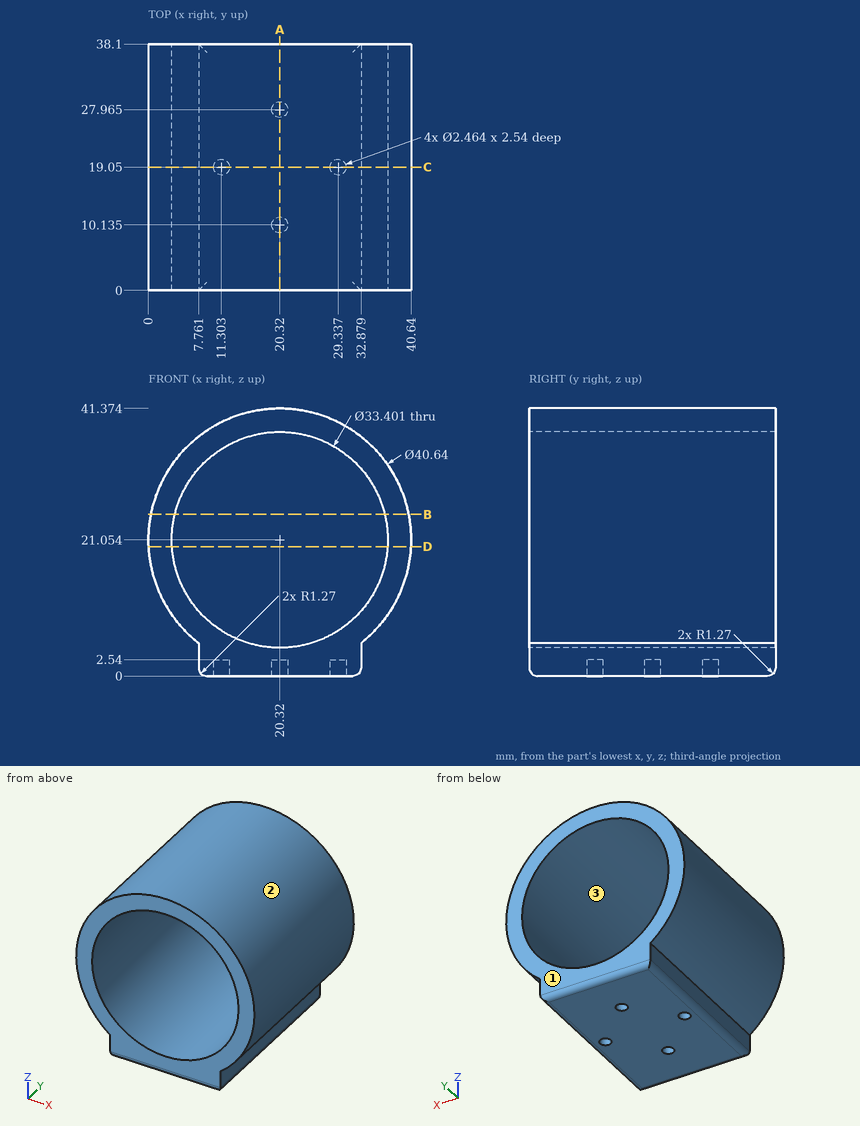
The figure shows three views and two pictorial views of one solid part (mm, origin at its lowest corner). Answer the questions. Give positions to 0.01 mm unless a question says otherwise; leave off trailing zeros. Write each loop counter-clockwise with the first axis right and the second up, starting at its lowest first coordinate (ties: lowest second). Pieces come first, ordered by that corner, then holes. Notation, with made-up numbers: M 35.5,66 L 58.5,66 A20 ccw 58.5,96 Z; hole C 54.5,-7.5 d1. An arc over 180 degrees is marked long. One line per item, written item: value. Start each with the question number.
(1) Find the intervals of material crossed by line 1 (Z direction, x = 20, y = 30); line 2 (Z direction, x = 22, y = 18) (1 decimal); line 3 (X direction, y = 22.5, z = 33), in increasing order.
(2) Find section A-A (x = 20.32). Determine the outline of the cut face in (y, z) (1 decimal).
(3) Determine the mould class of the marked faces 1, 2 and 3 for opening direction Z: pulls with the +Z half, pulls with the -Z half, needs draft (parallel to the pull), parting line crosses it, or undercut.
(4) Find section C-C (y = 19.05). Determine the outline of the cut face in (x, z) (1 decimal), plus the area to 3 significant figures.
(5) Flat-ended cylindrical pins translate along their axes: pin 1 Ø1 at (x, y) = (8.5, 7.5) entering from +Z; pin 2 Ø3 at (y, z) = (21.5, 19) entering from +X; pin 3 Ø2 at (x, y) = (20.32, 27.97) entering from -Z; pin 4 Ø2.5 at (x, y) = (29, 19) entering from -Z. Find the tip coordinate at first contact, or state that the pin passes through.
(6) Find section B-B (z = 25). Determine the outline of the cut face in (x, y), plus the area to 3 significant figures.
(7) Find section D-D (z = 20). Determine the outline of the cut face in (x, y), plus the area to 3 significant figures.
Results below:
1. line 1: z = 0 to 4.36, 37.75 to 41.37
1. line 2: z = 0 to 4.4, 37.7 to 41.3
1. line 3: x = 3.88 to 8.65, 31.99 to 36.76
2. outline: M 0,1.3 A1.3 ccw 1.3,0 L 8.9,0 L 8.9,2.5 L 11.4,2.5 L 11.4,0 L 26.7,0 L 26.7,2.5 L 29.2,2.5 L 29.2,0 L 36.8,0 A1.3 ccw 38.1,1.3 L 38.1,4.4 L 0,4.4 Z; M 0,37.8 L 38.1,37.8 L 38.1,41.4 L 0,41.4 Z
3. face 1: needs draft
3. face 2: parting line crosses it
3. face 3: undercut
4. outline: M 7.8,1.3 A1.3 ccw 9,0 L 10.1,0 L 10.1,2.5 L 12.5,2.5 L 12.5,0 L 28.1,0 L 28.1,2.5 L 30.6,2.5 L 30.6,0 L 31.6,0 A1.3 ccw 32.9,1.3 L 32.9,5.1 A20.3 ccw long 7.8,5.1 Z; hole C 20.3,21.1 d33.4
4. area: 461 mm^2
5. pin 1: stops at z = 37.93
5. pin 2: stops at x = 40.63
5. pin 3: stops at z = 2.54
5. pin 4: stops at z = 0
6. outline: M 0.39,0 L 4.09,0 L 4.09,38.1 L 0.39,38.1 Z; M 36.55,0 L 40.25,0 L 40.25,38.1 L 36.55,38.1 Z
6. area: 282 mm^2
7. outline: M 0.03,0 L 3.65,0 L 3.65,38.1 L 0.03,38.1 Z; M 36.99,0 L 40.61,0 L 40.61,38.1 L 36.99,38.1 Z
7. area: 276 mm^2
